from build123d import *

# Parameters (mm, degrees)
ESQUISSE1_R        = 3.5
ESQUISSE1_R_2      = 4
ESQUISSE1_R_3      = 5.75
ESQUISSE1_R_4      = 4.5
ESQUISSE1_W        = 81
ESQUISSE1_H        = 51.2
BOSS_EXTRU_1_DEPTH = 3
ESQUISSE2_W        = 7.242640687
ESQUISSE2_H        = 7.242640687
ESQUISSE2_R        = 1.965304202
ESQUISSE2_R_2      = 2
ESQUISSE2_R_3      = 2.113486369
BOSS_EXTRU_2_DEPTH = 3


with BuildPart() as part:
    # Esquisse1 → Boss.-Extru.1 (new body)
    with BuildSketch(Plane.XY.offset(0.8)):
        with BuildLine():
            Line((-112.589634865, 39.905491149), (24.864852981, 39.905491149))
            Line((24.864852981, 39.905491149), (24.864852981, 35.662850462))
            ThreePointArc((24.864852981, 35.662850462), (25.743532637, 33.541530119), (27.864852981, 32.662850462))
            Line((27.864852981, 32.662850462), (32.107493668, 32.662850462))
            Line((32.107493668, 32.662850462), (32.107493668, -31.368742114))
            Line((32.107493668, -31.368742114), (27.864852981, -31.368742114))
            ThreePointArc((27.864852981, -31.368742114), (25.743532637, -32.24742177), (24.864852981, -34.368742114))
            Line((24.864852981, -34.368742114), (24.864852981, -38.611382801))
            Line((24.864852981, -38.611382801), (-112.589634865, -38.611382801))
            Line((-112.589634865, -38.611382801), (-112.589634865, -34.368742114))
            ThreePointArc((-112.589634865, -34.368742114), (-113.468314521, -32.24742177), (-115.589634865, -31.368742114))
            Line((-115.589634865, -31.368742114), (-119.832275552, -31.368742114))
            Line((-119.832275552, -31.368742114), (-119.832275552, 32.662850462))
            Line((-119.832275552, 32.662850462), (-115.589634865, 32.662850462))
            ThreePointArc((-115.589634865, 32.662850462), (-113.468314521, 33.541530119), (-112.589634865, 35.662850462))
            Line((-112.589634865, 35.662850462), (-112.589634865, 39.905491149))
        make_face()
        with Locations((-109.194417438, 24.821428571)):
            Circle(ESQUISSE1_R, mode=Mode.SUBTRACT)
        with Locations((-1.194417438, 24.821428571)):
            Circle(ESQUISSE1_R, mode=Mode.SUBTRACT)
        with Locations((-1.194417438, -21.178571429)):
            Circle(ESQUISSE1_R, mode=Mode.SUBTRACT)
        with Locations((-109.194417438, -21.178571429)):
            Circle(ESQUISSE1_R, mode=Mode.SUBTRACT)
        with Locations((14.345224597, 6.749852674)):
            Circle(ESQUISSE1_R_2, mode=Mode.SUBTRACT)
        with Locations((5.845224597, 16.204342535)):
            Circle(ESQUISSE1_R, mode=Mode.SUBTRACT)
        with Locations((22.845224597, 16.204342535)):
            Circle(ESQUISSE1_R, mode=Mode.SUBTRACT)
        with Locations((22.845224597, -6.795657465)):
            Circle(ESQUISSE1_R, mode=Mode.SUBTRACT)
        with Locations((5.845224597, -6.795657465)):
            Circle(ESQUISSE1_R, mode=Mode.SUBTRACT)
        with Locations((14.176552179, -18.611382801)):
            Circle(ESQUISSE1_R_3, mode=Mode.SUBTRACT)
        with Locations((-35.905557573, -31.316718293)):
            Circle(ESQUISSE1_R_4, mode=Mode.SUBTRACT)
        with Locations((-79.237508709, -31.316718293)):
            Circle(ESQUISSE1_R_4, mode=Mode.SUBTRACT)
        with Locations((-55.194417438, 1.821428571)):
            Rectangle(ESQUISSE1_W, ESQUISSE1_H, mode=Mode.SUBTRACT)
    extrude(amount=BOSS_EXTRU_1_DEPTH)

    # Esquisse2 → Boss.-Extru.2 (add)
    # profile 1 of 4: a face of its own
    with BuildSketch(Plane.XY.offset(0.8)):
        with Locations((-116.210955209, -34.990062458)):
            Rectangle(ESQUISSE2_W, ESQUISSE2_H)
        with Locations((-116.210955208, -34.990062458)):
            Circle(ESQUISSE2_R, mode=Mode.SUBTRACT)
    # profile 2 of 4: a face of its own
    with BuildSketch(Plane.XY.offset(0.8)):
        with Locations((-116.210955209, 36.284170805)):
            Rectangle(ESQUISSE2_W, ESQUISSE2_H)
        with Locations((-116.210955208, 36.284170806)):
            Circle(ESQUISSE2_R_2, mode=Mode.SUBTRACT)
    # profile 3 of 4: a face of its own
    with BuildSketch(Plane.XY.offset(0.8)):
        with Locations((28.486173325, 36.284170805)):
            Rectangle(ESQUISSE2_W, ESQUISSE2_H)
        with Locations((28.486173324, 36.284170806)):
            Circle(ESQUISSE2_R_3, mode=Mode.SUBTRACT)
    # profile 4 of 4: a face of its own
    with BuildSketch(Plane.XY.offset(0.8)):
        with Locations((28.486173325, -34.990062458)):
            Rectangle(ESQUISSE2_W, ESQUISSE2_H)
        with Locations((28.486173324, -34.990062458)):
            Circle(ESQUISSE2_R_2, mode=Mode.SUBTRACT)
    extrude(amount=BOSS_EXTRU_2_DEPTH)


solid = part.part
Read the model definition and answer for the solid it produces. Units are mm, in the model's axes. A direction names the side the tool comes from. Coordinates: 2 decimals unless noted, no trailing zeros. Write each loop counter-clockwise with the first axis right and the second up, starting at its lowest first coordinate (ties: lowest second). Pieces come first, ordered by that corner, then holes. Notation, with made-up numbers: M -8,39 L 30,39 A13 ccw 30,58 Z; hole C -32,0.25 d3. An arc over 180 degrees is marked long. Use a Markdown table: item, result.
Q1. The part is cut by section A-A, the plane z = 3.15. Give the number of separate pieces and of enclosed holes in the cut face, then the cut area to 3 significant figures.
Answer block:
| item | result |
|---|---|
| separate pieces | 1 |
| enclosed holes | 17 |
| area | 7,140 mm2 |
Q2. This flat-tipped pin is pushed along its axis until it touches: pin 1 Ø7 at (x, y) = (14.18, -18.61) entering from -Z. Where does it stop, or does it pass through?
Answer block:
| item | result |
|---|---|
| pin 1 | passes through |
Q3. Straight lines are drawn through the part: L1, parallel to Y at x = -48, z = 3.5; L2, parallel to X at y = -22.5, z = 2.25; L3, parallel to Y at x = -37, z = 1.45. For each, find the intervals that lie inside material, in ascending order. Write a range as [from, to].
Answer block:
| item | result |
|---|---|
| L1 | y = [-38.61, -23.78], [27.42, 39.91] |
| L2 | x = [-119.83, -112.44], [-105.95, -95.69], [-14.69, -4.44], [2.05, 9.94], [18.41, 32.11] |
| L3 | y = [-38.61, -35.68], [-26.95, -23.78], [27.42, 39.91] |
Q4. Determine the mould class of faces 3 (the face through (-56, -23.779, 2)), 4 (the face through (-119.832, 0, 2)), 5 (the face through (32.107, 1, 2)) for opening direction X: released by +X, released by -X, zero draft, split by the parting line, or undercut.
Answer block:
| item | result |
|---|---|
| face 3 | undercut |
| face 4 | released by -X |
| face 5 | released by +X |
Q5. The part is cut by section B-B, the plane y = 14.5. Write down the section's boundary in (x, z), then the cut area to 3 significant figures.
Answer block:
| item | result |
|---|---|
| outline | M -119.83,0.8 L -95.69,0.8 L -95.69,3.8 L -119.83,3.8 Z; M -14.69,0.8 L 2.79,0.8 L 2.79,3.8 L -14.69,3.8 Z; M 8.9,0.8 L 19.79,0.8 L 19.79,3.8 L 8.9,3.8 Z; M 25.9,0.8 L 32.11,0.8 L 32.11,3.8 L 25.9,3.8 Z |
| area | 176 mm2 |
Q6. Which of the six approach directions +Z, -Z, +X, -X, +Y, -Y give full straight-line access (tool end or side, diameter ignored) to faces 1 (the face through (-95.694, 1, 2)), 2 (the face through (-45, -25, 3.8))?
Answer block:
| item | result |
|---|---|
| face 1 | +Z, -Z |
| face 2 | +Z, +X, -X, +Y, -Y |
